The drawing under review shows one solid part. Ordinate dimensions are in mm from its lowest x, y, z. A direction names the side the tool comes from. Round coordinates to 2 decimals unless told otherwise and drop trailing zeros. Write each loop counter-clockwise with the first axis right and the second up, starting at its lowest first coordinate (ties: lowest second). Pieces come first, ordered by that corner, then holes.
Item 1: Machinability: for the marked faces 1, 2, 3, 4 and 5, which of the approach directions +Z, -Z, +X, -X, +Y, -Y give a long, thin tool a straight path to every point of the face, cutting with its end or side? Answer none if there is none.
Item 2: Add section D-D (y = 12). Give the boundary of the cut face in (x, z), plus the area to 3 significant figures.
Item 3: Add section A-A (z = 65). Give the boundary of the cut face in (x, y).
Item 4: To check wall thickness, follow L1, parallel to Z at x = 1.05, y = 7.5; L2, parallel to Y at x = 16, z = 17; L3, parallel to X at y = 8, z = 58.5. State the ranges of each line that lie inside material, in increasing order.
Item 5: Add section B-B (y = 7.5). Give the boundary of the cut face in (x, z), plus the area to 3 significant figures.
Item 6: Add section C-C (x = 1). Give the boundary of the cut face in (y, z).
Item 7: Clearance check with flat-ended pins moving along their axes: pin 1 Ø10 at (x, z) = (11, 37.5) entering from -Y; pin 2 Ø3 at (y, z) = (12, 58.5) entering from +X; pin 3 Ø10 at (x, z) = (12, 37) entering from +Y. State where each tip first meets the part, or that it passes through.
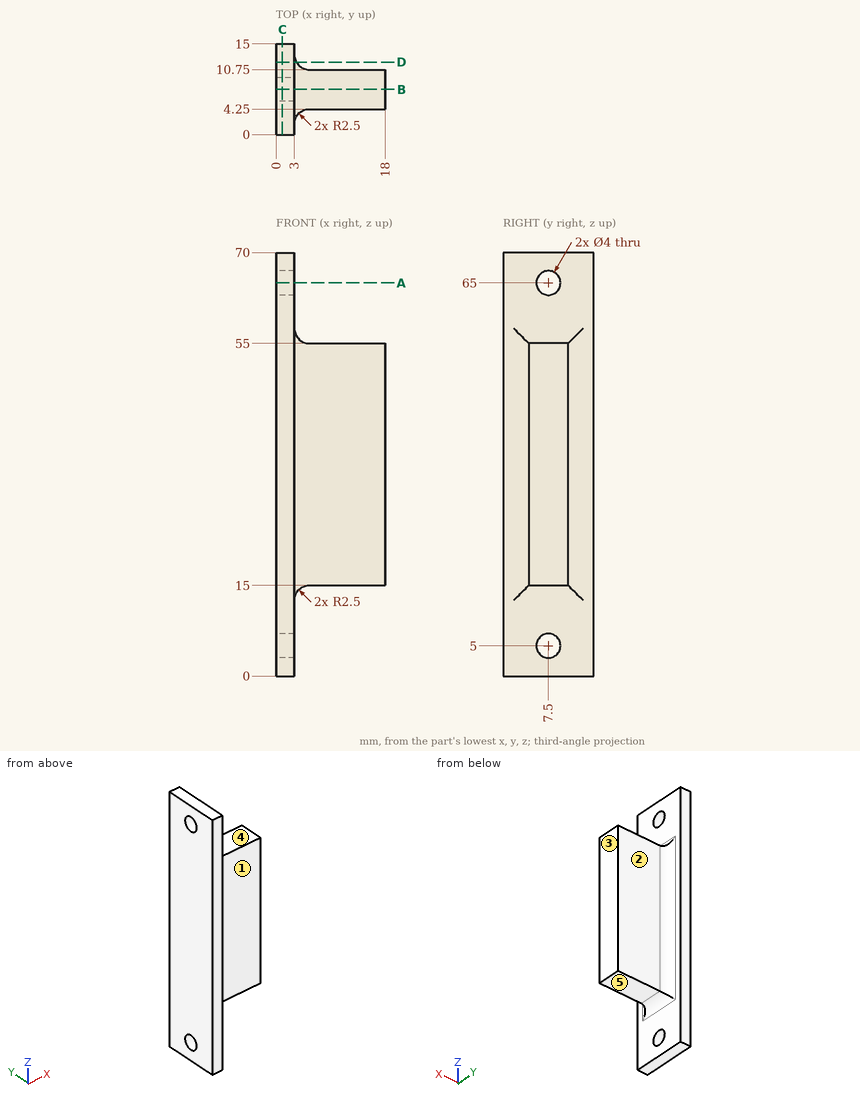
Numbers:
1. face 1: +Z, -Z, +X, -Y
1. face 2: +Z, -Z, +X, +Y
1. face 3: +Z, -Z, +X, +Y, -Y
1. face 4: +Z, +X, +Y, -Y
1. face 5: -Z, +X, +Y, -Y
2. outline: (0, 0) - (3, 0) - (3, 12.5) arc R2.5 cw to (3.33, 13.75) - (3.33, 56.25) arc R2.5 cw to (3, 57.5) - (3, 70) - (0, 70) - close
2. area: 225 mm2
3. outline: (0, 0) - (3, 0) - (3, 5.5) - (0, 5.5) - close; (0, 9.5) - (3, 9.5) - (3, 15) - (0, 15) - close
4. L1: z = 0 to 3, 7 to 63, 67 to 70
4. L2: y = 4.25 to 10.75
4. L3: x = 0 to 3
5. outline: (0, 0) - (3, 0) - (3, 3) - (0, 3) - close; (0, 7) - (3, 7) - (3, 12.5) arc R2.5 cw to (5.5, 15) - (18, 15) - (18, 55) - (5.5, 55) arc R2.5 cw to (3, 57.5) - (3, 63) - (0, 63) - close; (0, 67) - (3, 67) - (3, 70) - (0, 70) - close
5. area: 789 mm2
6. outline: (0, 0) - (15, 0) - (15, 70) - (0, 70) - close; hole circle Ø4 at (7.5, 5); hole circle Ø4 at (7.5, 65)
7. pin 1: stops at y = 4.25
7. pin 2: stops at x = 3.05
7. pin 3: stops at y = 10.75
